Geometry check sheet. Reference: the model listing, model coordinates, mm. Give positions to 0.01 mm unless a question says otherwise; leave off trailing zeros. Write each loop counter-clockwise with the first axis right and the second up, starting at its lowest first coordinate (ties: lowest second). Pieces come first, ordered by that corner, then holes. Notation, with made-up numbers: M 49,9 L 71,9 A21 cw 71,42 Z; hole C -3,0 d2. An arc over 180 degrees is marked long. One line per item, written item: value. Start each with the question number.
1. Gauge pin test, flat ends, axial feed: pin 1 (2 mm diameter, centred on x = 77.5, z = -11.5, fed in from -Y); pin 2 (10 mm diameter, centred on y = -4, z = 23, fed in from +X); pin 3 (12 mm diameter, centred on x = 10.5, y = 22, fed in from -Z); pin 4 (4 mm diameter, centred on x = 93.99, y = -1.22, fed in from +Z). Record the tip position at first contact, or that the pin passes through.
2. Cross-section at D-D on z = -2.5. Record the cut outline in (x, y).
3. Scan lines: line 1 (X direction, y = 6.5, z = 26); line 2 (X direction, y = 19.5, z = -1); line 3 (Z direction, x = 64, y = 0). Record each from-to range of solid material in increasing order.
4. Cross-section at A-A on z = 10. Record the cut outline in (x, y).
5. Cross-section at C-C on z = -19.5. Record the cut outline in (x, y), then the cut area to 3 significant figures.
6. Cross-section at B-B on y = -14. Record the cut outline in (x, z).
7. Release check for a two-part mould opening along Y. For faces 1 (the face through (56.53, 14.93, 6.09)), 2 (the face through (8.837, -5.301, -26.095)), 3 (the face through (12.7, 8, 16)), 4 (the face through (8.837, 5.788, 29.017)) record: pulls with the +Y half, pulls with the -Y half, needs draft (parallel to the pull), parting line crosses it, or undercut.
from build123d import *

# Parameters (mm, degrees)
F0_R          = 15.399925
F1_DEPTH      = 101.6
F2_R          = 15.399925
F3_DEPTH      = 12.7
F4_SIZE       = 5.08
F5_R          = 3.511723
F6_DEPTH      = 32.301025
F6_DEPTH_BACK = 29.379094


with BuildPart() as f1:
    # F0 (on Right) → F1 (new body)
    with BuildSketch(Plane.YZ):
        with Locations((0.243489, 1.460966)):
            Circle(F0_R)
    extrude(amount=F1_DEPTH)

    # F2 (on face) → F3 (join)
    with BuildSketch(Plane(origin=(0, 0, 0), x_dir=(0, -1, 0), z_dir=(-1, 0, 0))):
        Polygon((31.521783, 8.120019), (9.872238, 32.300025), (-21.893034, 25.640972), (-32.008761, -5.198088), (-10.359216, -29.378094), (21.406057, -22.71904), align=None)
        with Locations((-0.243489, 1.460966)):
            Circle(F2_R, mode=Mode.SUBTRACT)
    extrude(amount=-F3_DEPTH)

    # F4
    f4_edges = [f1.edges().sort_by_distance(p)[0] for p in [
        (0, 26.950898, 10.221442),
        (0, 6.010398, 28.970498),
        (0, -20.697011, 20.210022),
        (0, -26.46392, -7.299511),
        (0, -5.52342, -26.048567),
        (0, 21.183988, -17.288091),
    ]]
    chamfer(f4_edges, length=F4_SIZE)

    # F5 (on Top) → F6 (cut, two sides)
    with BuildSketch(Plane.XY) as f6_sk:
        with Locations((93.988761, -1.217474)):
            Circle(F5_R)
    extrude(amount=F6_DEPTH, mode=Mode.SUBTRACT)
    extrude(f6_sk.sketch, amount=-F6_DEPTH_BACK, mode=Mode.SUBTRACT)


solid = f1.part
Report:
1. pin 1: stops at y = -9.46
1. pin 2: stops at x = 12.7
1. pin 3: stops at z = -23.08
1. pin 4: passes through
2. outline: M 0,-22.69 L 5.08,-28.04 L 12.7,-28.04 L 12.7,-14.64 L 101.6,-14.64 L 101.6,15.13 L 12.7,15.13 L 12.7,31.12 L 5.08,31.12 L 0,25.78 Z; hole C 93.99,-1.22 d7.02
3. line 1: x = 2.27 to 12.7
3. line 2: x = 0 to 12.7
3. line 3: z = -13.94 to 16.86
4. outline: M 0,-23.02 L 5.08,-29.84 L 12.7,-29.84 L 12.7,-12.57 L 101.6,-12.57 L 101.6,13.06 L 12.7,13.06 L 12.7,27.02 L 5.08,27.02 L 0,21.68 Z; hole C 93.99,-1.22 d7.02
5. outline: M 0,-12 L 1.34,-18.52 L 5.08,-22.46 L 12.7,-22.46 L 12.7,19.2 L 5.08,19.2 L 0,12.38 Z
5. area: 495 mm^2
6. outline: M 0,-19.08 L 5.08,-24.27 L 12.7,-24.27 L 12.7,-4.39 L 101.6,-4.39 L 101.6,7.32 L 12.7,7.32 L 12.7,27.69 L 5.08,27.69 L 0,20.07 Z
7. face 1: parting line crosses it
7. face 2: pulls with the -Y half
7. face 3: needs draft
7. face 4: pulls with the +Y half
